Autodesk Inventor part; units mm, degrees
ref_plane "YZ Plane" through (0, 0, 0) normal (1, 0, 0) x (0, 1, 0)
ref_plane "XZ Plane" through (0, 0, 0) normal (0, 1, 0) x (-1, 0, 0)
ref_plane "XY Plane" through (0, 0, 0) normal (0, 0, 1) x (1, 0, 0)
sketch "Sketch1" plane through (0, 0, 0) normal (0, 0, 1) x (1, 0, 0)
  line L0 (0, 0) -> (-177.8, 0)
  line L1 (-177.8, 0) -> (-177.8, 88.9)
  line L2 (0, 0) -> (0, 88.9)
  line L3 (2.54, 88.9) -> (2.54, -2.54)
  line L4 (2.54, -2.54) -> (-180.34, -2.54)
  line L5 (-180.34, -2.54) -> (-180.34, 88.9)
  line L6 (-180.34, 88.9) -> (-177.8, 88.9)
  line L7 (2.54, 88.9) -> (0, 88.9)
  dimension "d0" = 177.8
  dimension "d2" = 2.54
  dimension "d13" = 88.9
extrude "Extrusion1" add sketch "Sketch1" along normal blind 171.45
sketch "Sketch2" plane through (2.54, -2.54, 0) normal (1, 0, 0) x (0, 0, -1)
  line L0 (0, 0) -> (0, 91.44)
  line L1 (0, 0) -> (2.54, 0)
  line L2 (2.54, 0) -> (2.54, 91.44)
  line L3 (2.54, 91.44) -> (0, 91.44)
  line L4 (0, 91.44) -> (0, 0)
  point P0 (0, 2.54)
  point P1 (1.27, 91.44)
  dimension "d5" = 2.54
extrude "Extrusion2" add sketch "Sketch2" against normal up to surface (182.88 mm away)
sketch "Sketch3" plane through (-177.8, 0, 0) normal (0, 0, 1) x (1, 0, 0)
  line L0 (56.6436, 81.28) -> (121.1564, 81.28) construction
  line L1 (59.1836, 78.74) -> (118.6164, 78.74)
  line L2 (118.6164, 83.82) -> (59.1836, 83.82)
  arc A0 (59.1836, 83.82) -> (59.1836, 78.74) centre (59.1836, 81.28) ccw
  arc A1 (118.6164, 78.74) -> (118.6164, 83.82) centre (118.6164, 81.28) ccw
  line L3 (177.8, 88.9) -> (0, 88.9)
  line L4 (177.8, 0) -> (0, 0)
  point P0 (88.9, 81.28)
  point P1 (88.9, 83.82)
  point P2 (88.9, 88.9)
  dimension "d9" = 5.08
  dimension "d10" = 81.28
extrude "Extrusion3" cut sketch "Sketch3" against normal through all
properties part number "batteryholder-ver1-1111-2017"
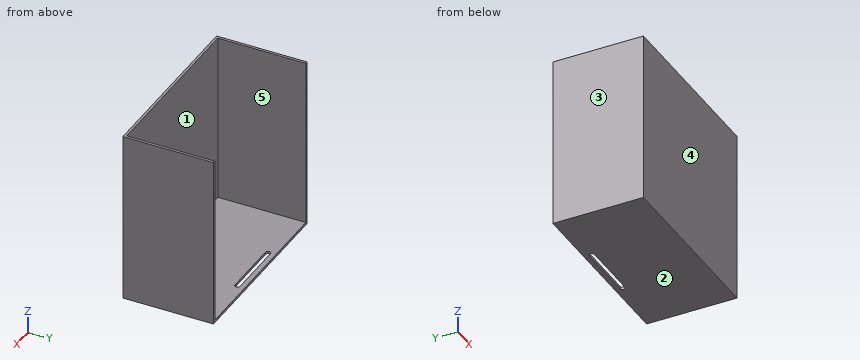
Source: CAD feature listing. Evaluate the final solid. Frame: model axes, mm. Face numbers are marked on the shaded views. A direction names the side the tool comes from. Give positions to 0.01 mm unless a question says otherwise; leave off trailing zeros. Order: outer loops, then holes, each group sorted by start corner. A loop starts at its lowest first (then second) coordinate and runs counter-clockwise, first axis right, second up.
(1) Access query for the marked faces 1 and 2. Directions: +Z, -Z, +X, -X, +Y, -Y. A direction counts if a zero-diameter tool reaches every point of the face in a straight line with its end or side. Return the directions, or none.
(2) Pull-direction query (X, two-part tool) for the marked faces 3, 4 and 5; classes: +X half, -X half, draft (parallel to the pull), parting line (faces both ways), or undercut.
(3) Section query D-D (y = 38). Return the cut outline in (x, z), plus the area to 3 significant figures.
(4) Section query C-C (z = 112). Return the cut outline in (x, y), plus the area to 3 significant figures.
(5) Section query B-B (y = 81.28). Return the cut outline in (x, z), plus the area to 3 significant figures.
(6) Contact query for a flat-ended pin moving along its axis: P1, Ø3, axis at x = -50, y = 59, coming from the +Z side. Output: stop coordinate, or through.
(7) Material intervals for line 1 along X through (y, z) = (25.5, 156); line 2 along Z through (x, y) = (-152, 71), sorted ascending.
(8) Section query A-A (x = -72). Return the cut outline in (y, z), plus the area to 3 significant figures.
Outcome:
1. face 1: +Z, +Y
1. face 2: -Z, +X, -X, +Y, -Y
2. face 3: -X half
2. face 4: draft
2. face 5: undercut
3. outline: (-180.34, -2.54) - (2.54, -2.54) - (2.54, 171.45) - (0, 171.45) - (0, 0) - (-177.8, 0) - (-177.8, 171.45) - (-180.34, 171.45) - close
3. area: 1,340 mm2
4. outline: (-180.34, -2.54) - (2.54, -2.54) - (2.54, 88.9) - (0, 88.9) - (0, 0) - (-177.8, 0) - (-177.8, 88.9) - (-180.34, 88.9) - close
4. area: 916 mm2
5. outline: (-180.34, -2.54) - (-121.16, -2.54) - (-121.16, 0) - (-177.8, 0) - (-177.8, 171.45) - (-180.34, 171.45) - close; (-56.64, -2.54) - (2.54, -2.54) - (2.54, 171.45) - (0, 171.45) - (0, 0) - (-56.64, 0) - close
5. area: 1,170 mm2
6. P1: stops at z = 0
7. line 1: x = -180.34 to -177.8, 0 to 2.54
7. line 2: z = -2.54 to 0
8. outline: (-2.54, -2.54) - (78.74, -2.54) - (78.74, 0) - (0, 0) - (0, 171.45) - (-2.54, 171.45) - close; (83.82, -2.54) - (88.9, -2.54) - (88.9, 0) - (83.82, 0) - close
8. area: 655 mm2
